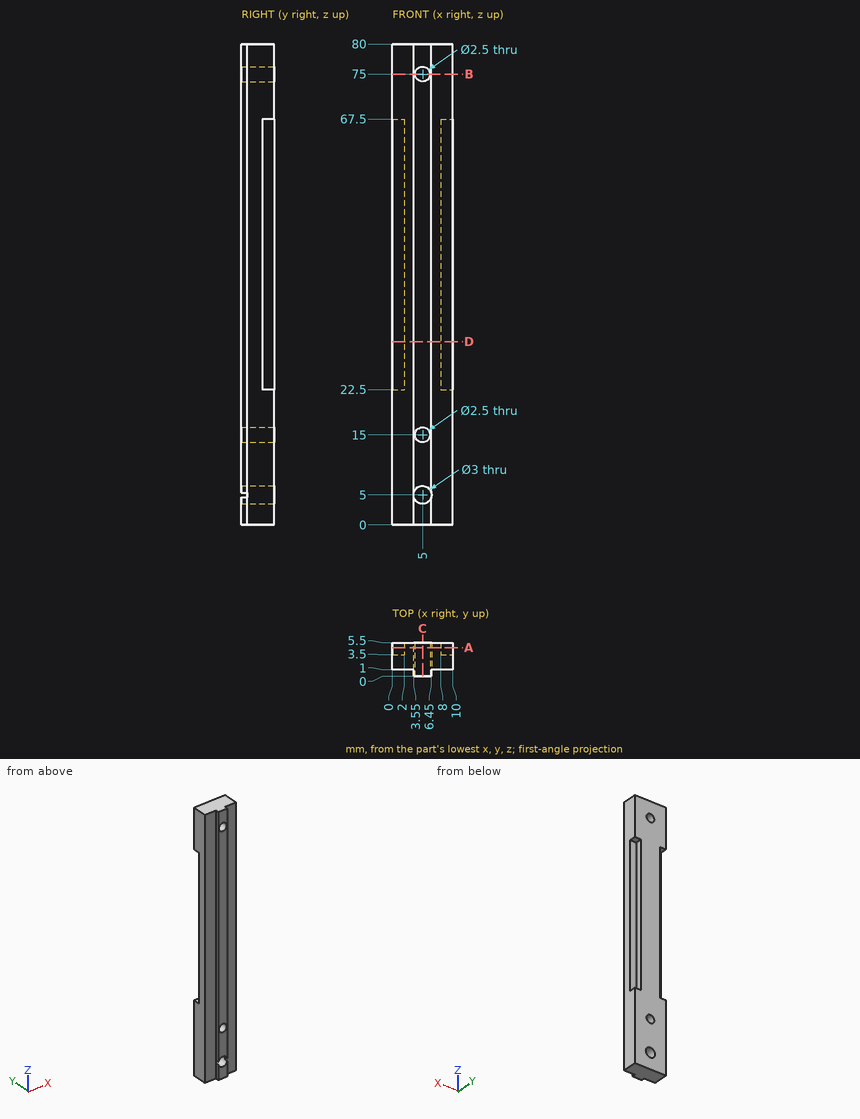
For this review, use the dimensioned drawing (mm, ordinates from the lowest corner) and the shaded views. Round coordinates to 2 decimals unless told otherwise and drop trailing zeros. Order: outer loops, then holes, each group sorted by start corner. A loop starts at its lowest first (then second) coordinate and runs counter-clockwise, first axis right, second up. Notation, with made-up numbers: (51.5, 58.25) -> (59.5, 58.25) arc R27 ccw to (59.5, 79.25) -> close; hole circle Ø7 at (16.5, 28). An arc over 180 degrees is marked (long way). Write item = value, one per line. Start each with the question number.
Item 1: Consider section D-D on z = 30.5. Write out the cut boundary in (x, y), plus the area to 3 significant figures.
Item 2: Consider section C-C on x = 5. Write out the cut boundary in (y, z), plus the area to 3 significant figures.
Item 3: For line 1 along Z through (x, y) = (5, 3.35); line 2 along Z through (x, y) = (0.75, 3.95); line 3 along X through (y, z) = (3.2, 75), list the stretches that pass through material, from the lowest coordinate up.
Item 4: Clearance check with flat-ended pins moving along their axes: pin 1 Ø1.6 at (y, z) = (4, 50) entering from +X; pin 2 Ø0.8 at (y, z) = (0.5, 56.5) entering from -X; pin 3 Ø2.5 at (x, z) = (5, 5) entering from +Y; pin 4 Ø1.8 at (x, z) = (1.5, 28) entering from -Y. State where each tip first meets the part, or that it passes through.
Item 5: Consider section B-B on z = 75. Write out the cut boundary in (x, y), plus the area to 4 significant figures.
Item 6: Consider section A-A on y = 4.7. Write out the cut boundary in (x, z), plus the area to 3 significant figures.
Conclusion:
q1.outline = (0, 1) -> (3.55, 1) -> (3.55, 0) -> (6.45, 0) -> (6.45, 1) -> (10, 1) -> (10, 3.5) -> (8, 3.5) -> (8, 5.5) -> (2, 5.5) -> (2, 3.5) -> (0, 3.5) -> close
q1.area = 39.9 mm2
q2.outline = (0, 0) -> (5.5, 0) -> (5.5, 3.5) -> (0, 3.5) -> close; (0, 6.5) -> (5.5, 6.5) -> (5.5, 13.75) -> (0, 13.75) -> close; (0, 16.25) -> (5.5, 16.25) -> (5.5, 73.75) -> (0, 73.75) -> close; (0, 76.25) -> (5.5, 76.25) -> (5.5, 80) -> (0, 80) -> close
q2.area = 396 mm2
q3.line_1 = 0 to 3.5, 6.5 to 13.75, 16.25 to 73.75, 76.25 to 80
q3.line_2 = 0 to 22.5, 67.5 to 80
q3.line_3 = 0 to 3.75, 6.25 to 10
q4.pin_1 = 10
q4.pin_2 = 3.55
q4.pin_3 = through
q4.pin_4 = 1
q5.outline = (0, 1) -> (3.55, 1) -> (3.55, 0) -> (3.75, 0) -> (3.75, 5.5) -> (0, 5.5) -> close; (6.25, 0) -> (6.45, 0) -> (6.45, 1) -> (10, 1) -> (10, 5.5) -> (6.25, 5.5) -> close
q5.area = 34.15 mm2
q6.outline = (0, 0) -> (10, 0) -> (10, 22.5) -> (8, 22.5) -> (8, 67.5) -> (10, 67.5) -> (10, 80) -> (0, 80) -> (0, 67.5) -> (2, 67.5) -> (2, 22.5) -> (0, 22.5) -> close; hole circle Ø3 at (5, 5); hole circle Ø2.5 at (5, 15); hole circle Ø2.5 at (5, 75)
q6.area = 603 mm2
